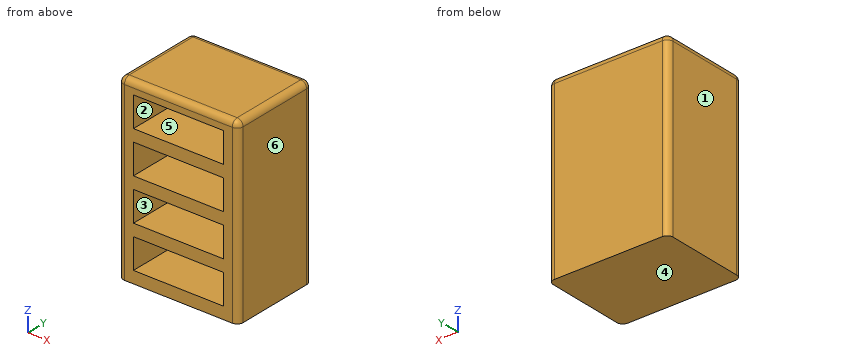
from build123d import *

# Parameters (mm, degrees)
F0_W     = 101.6
F0_H     = 76.2
F1_DEPTH = 152.4
F2_W     = 76.2
F2_H     = 25.4
F3_DEPTH = 50.8
F4_R     = 5.08


with BuildPart() as f1:
    # F0 (on Top) → F1 (new body)
    with BuildSketch(Plane.XY):
        with Locations((0.55306, -0.46621)):
            Rectangle(F0_W, F0_H)
    extrude(amount=F1_DEPTH)

    # F2 (on face) → F3 (cut)
    with BuildSketch(Plane.XZ.offset(38.56621)):
        with Locations((0.55306, 93.98)):
            Rectangle(F2_W, F2_H)
        with Locations((0.55306, 129.54)):
            Rectangle(F2_W, F2_H)
        with Locations((0.55306, 58.42)):
            Rectangle(F2_W, F2_H)
        with Locations((0.55306, 22.86)):
            Rectangle(F2_W, F2_H)
    extrude(amount=-F3_DEPTH, mode=Mode.SUBTRACT)

    # F4
    f4_edges = [f1.edges().sort_by_distance(p)[0] for p in [
        (51.35306, -0.46621, 152.4),
        (-50.24694, -0.46621, 152.4),
        (0.55306, -38.56621, 152.4),
        (0.55306, 37.63379, 152.4),
        (51.35306, -38.56621, 76.2),
        (-50.24694, -38.56621, 76.2),
        (51.35306, 37.63379, 76.2),
        (-50.24694, 37.63379, 76.2),
    ]]
    fillet(f4_edges, radius=F4_R)


solid = f1.part
Verification items for the finished model (mm, model axes). Face numbers are marked on the shaded views. A direction names the side the tool comes from. Coordinates: 2 decimals unless noted, no trailing zeros. Order: outer loops, then holes, each group sorted by start corner. A loop starts at its lowest first (then second) coordinate and runs counter-clockwise, first axis right, second up. Notation, with made-up numbers: (-27.75, 25) -> (-17.75, 25) arc R10 ccw to (-17.75, 34) -> close; hole circle Ø4 at (37, 76). An arc over 180 degrees is marked (long way). Put each result on its own line as item: value. Start each with the question number.
1. Access from +Z, -Z, +X, -X, +Y, -Y to the whole of each face (thin tool, end or side, straight path). Record for the marked faces 5 and 6.
2. Cross-section at B-B, the plane y = -13. Record the boundary of the cut face in (x, z), then the cut area to 3 significant figures.
3. Cross-section at C-C, the plane z = 91. Record the boundary of the cut face in (x, y).
4. Mould release check, pull along Z, two halves, no side actions. Record for the marked faces 1, 2, 3 and 4: released by +Z, released by -Z, zero draft, split by the parting line, or undercut.
5. Go/stop test with a flat-tipped pin: pin 1 Ø4 at (x, z) = (-7, 124) entering from -Y. Record where the tip stops, or that it passes through.
6. Cross-section at A-A, the plane x = 16.5. Record the boundary of the cut face in (y, z).
7. Material ranges on L1, parallel to Z at x = -4, y = -14; L2, parallel to X at y = -12.5, z = 132.5; L3, parallel to X at y = -34, z = 128, recorded low to high. Write a range as [from, to].
Computed:
1. face 5: -Y
1. face 6: +Z, -Z, +X, +Y, -Y
2. outline: (-50.25, 0) -> (51.35, 0) -> (51.35, 147.32) arc R5.08 ccw to (46.27, 152.4) -> (-45.17, 152.4) arc R5.08 ccw to (-50.25, 147.32) -> close; hole (-37.55, 10.16) -> (38.65, 10.16) -> (38.65, 35.56) -> (-37.55, 35.56) -> close; hole (-37.55, 45.72) -> (38.65, 45.72) -> (38.65, 71.12) -> (-37.55, 71.12) -> close; hole (-37.55, 81.28) -> (38.65, 81.28) -> (38.65, 106.68) -> (-37.55, 106.68) -> close; hole (-37.55, 116.84) -> (38.65, 116.84) -> (38.65, 142.24) -> (-37.55, 142.24) -> close
2. area: 7,730 mm2
3. outline: (-50.25, -33.49) arc R5.08 ccw to (-45.17, -38.57) -> (-37.55, -38.57) -> (-37.55, 12.23) -> (38.65, 12.23) -> (38.65, -38.57) -> (46.27, -38.57) arc R5.08 ccw to (51.35, -33.49) -> (51.35, 32.55) arc R5.08 ccw to (46.27, 37.63) -> (-45.17, 37.63) arc R5.08 ccw to (-50.25, 32.55) -> close
4. face 1: zero draft
4. face 2: undercut
4. face 3: undercut
4. face 4: released by -Z
5. pin 1: y = 12.23
6. outline: (-38.57, 0) -> (37.63, 0) -> (37.63, 147.32) arc R5.08 ccw to (32.55, 152.4) -> (-33.49, 152.4) arc R5.08 ccw to (-38.57, 147.32) -> (-38.57, 142.24) -> (12.23, 142.24) -> (12.23, 116.84) -> (-38.57, 116.84) -> (-38.57, 106.68) -> (12.23, 106.68) -> (12.23, 81.28) -> (-38.57, 81.28) -> (-38.57, 71.12) -> (12.23, 71.12) -> (12.23, 45.72) -> (-38.57, 45.72) -> (-38.57, 35.56) -> (12.23, 35.56) -> (12.23, 10.16) -> (-38.57, 10.16) -> close
7. L1: [0, 10.16], [35.56, 45.72], [71.12, 81.28], [106.68, 116.84], [142.24, 152.4]
7. L2: [-50.25, -37.55], [38.65, 51.35]
7. L3: [-50.22, -37.55], [38.65, 51.33]
